Autodesk Inventor part; units mm, degrees
ref_plane "YZ Plane" through (0, 0, 0) normal (1, 0, 0) x (0, 1, 0)
ref_plane "XZ Plane" through (0, 0, 0) normal (0, 1, 0) x (-1, 0, 0)
ref_plane "XY Plane" through (0, 0, 0) normal (0, 0, 1) x (1, 0, 0)
sketch "Sketch1" plane through (0, 0, 0) normal (0, 0, 1) x (1, 0, 0)
  line L0 (22.5, -10) -> (-22.5, -10) construction
  line L1 (-22.5, -10) -> (-22.5, 10) construction
  line L2 (-22.5, 10) -> (22.5, 10) construction
  line L3 (22.5, 10) -> (22.5, -10) construction
  line L4 (22.5, -10) -> (-22.5, 10) construction
  line L5 (-22.5, -10) -> (22.5, 10) construction
  line L6 (-22.5, 13) -> (-22.5, 7) construction
  line L7 (-24.25, 13) -> (-24.25, 7)
  line L8 (-20.75, 7) -> (-20.75, 13)
  arc A0 (-20.75, 13) -> (-24.25, 13) centre (-22.5, 13) ccw
  arc A1 (-24.25, 7) -> (-20.75, 7) centre (-22.5, 7) ccw
  line L9 (-22.5, -13) -> (-22.5, -7) construction
  line L10 (-20.75, -13) -> (-20.75, -7)
  line L11 (-24.25, -7) -> (-24.25, -13)
  arc A2 (-24.25, -13) -> (-20.75, -13) centre (-22.5, -13) ccw
  arc A3 (-20.75, -7) -> (-24.25, -7) centre (-22.5, -7) ccw
  line L12 (22.5, 13) -> (22.5, 7) construction
  line L13 (20.75, 13) -> (20.75, 7)
  line L14 (24.25, 7) -> (24.25, 13)
  arc A4 (24.25, 13) -> (20.75, 13) centre (22.5, 13) ccw
  arc A5 (20.75, 7) -> (24.25, 7) centre (22.5, 7) ccw
  line L15 (22.5, -13) -> (22.5, -7) construction
  line L16 (24.25, -13) -> (24.25, -7)
  line L17 (20.75, -7) -> (20.75, -13)
  arc A6 (20.75, -13) -> (24.25, -13) centre (22.5, -13) ccw
  arc A7 (24.25, -7) -> (20.75, -7) centre (22.5, -7) ccw
  line L18 (26, -16.5) -> (-26, -16.5)
  line L19 (-26, -16.5) -> (-26, 16.5)
  line L20 (-26, 16.5) -> (26, 16.5)
  line L21 (26, 16.5) -> (26, -16.5)
  line L22 (26, -16.5) -> (-26, 16.5) construction
  line L23 (-26, -16.5) -> (26, 16.5) construction
  circle A8 centre (0, 0) radius 6.35
  dimension "d0" = 45
  dimension "d1" = 20
  dimension "d2" = 3.5
  dimension "d3" = 6
  dimension "d4" = 52
  dimension "d5" = 33
  dimension "d6" = 12.7
extrude "Extrusion1" add sketch "Sketch1" along normal blind 4.7625
fillet "Fillet1" radius 2 4 edges at (-26, 16.5, 2.3813) (26, 16.5, 2.3813) (26, -16.5, 2.3813) (-26, -16.5, 2.3813)
properties part number "belt tensioner"
Source: CAD feature listing. Evaluate the final solid. Frame: model axes, mm. A direction names the side the tool comes from. Coordinates: 2 decimals unless noted, no trailing zeros. Loops run counter-clockwise (first coordinate to the right, second up) from the corner with the lowest first, then second, coordinate; pieces in that order, holes last. Notation, with made-up numbers: (75.25, 73) - (104.25, 73) arc R18 ccw to (104.25, 95) - close; hole circle Ø6 at (72, 20). An arc over 180 degrees is marked (long way). One line per question, with ' | ' between items.
1) Line query: line 1 along X through (y, z) = (9.5, 3.6); line 2 along Y through (x, z) = (0, 1.55); line 3 along X through (y, z) = (14, 0.75). Output: solid intervals per line, ascending.
Report:
line 1: x = -26 to -24.25, -20.75 to 20.75, 24.25 to 26 | line 2: y = -16.5 to -6.35, 6.35 to 16.5 | line 3: x = -26 to -23.94, -21.06 to 21.06, 23.94 to 26
2) Section C-C, the plane z = 3.5. Return loops of the section in (x, y), then the cut area to 3 significant figures.
Report:
outline: (-26, -14.5) arc R2 ccw to (-24, -16.5) - (24, -16.5) arc R2 ccw to (26, -14.5) - (26, 14.5) arc R2 ccw to (24, 16.5) - (-24, 16.5) arc R2 ccw to (-26, 14.5) - close; hole (-24.25, -13) arc R1.75 ccw to (-20.75, -13) - (-20.75, -7) arc R1.75 ccw to (-24.25, -7) - close; hole (-24.25, 7) arc R1.75 ccw to (-20.75, 7) - (-20.75, 13) arc R1.75 ccw to (-24.25, 13) - close; hole circle Ø12.7 at (0, 0); hole (20.75, -13) arc R1.75 ccw to (24.25, -13) - (24.25, -7) arc R1.75 ccw to (20.75, -7) - close; hole (20.75, 7) arc R1.75 ccw to (24.25, 7) - (24.25, 13) arc R1.75 ccw to (20.75, 13) - close | area: 1,460 mm²
3) Pull-direction query (X, two-part tool) for faces 3 (the face through (-6, 4, 4.762)), 4 (the face through (20.75, 10, 2)), 5 (the face through (26, 0, 2)); classes: released by +X, released by -X, zero draft, split by the parting line, or undercut.
Report:
face 3: zero draft | face 4: undercut | face 5: released by +X
4) Set-up query: faces 1 (the face through (-24.25, -10, 2)), 2 (the face through (0, -16.5, 2)). Return all of +Z, -Z, +X, -X, +Y, -Y with unobstructed straight access to the full face (end or side cutting, diameter ignored); none if empty.
Report:
face 1: +Z, -Z | face 2: +Z, -Z, +X, -X, -Y
5) Section A-A, the plane x = 22.5. Return loops of the section in (y, z).
Report:
outline: (-16.5, 0) - (-14.75, 0) - (-14.75, 4.76) - (-16.5, 4.76) - close; (-5.25, 0) - (5.25, 0) - (5.25, 4.76) - (-5.25, 4.76) - close; (14.75, 0) - (16.5, 0) - (16.5, 4.76) - (14.75, 4.76) - close
6) Section B-B, the plane y = 0. Return loops of the section in (x, z).
Report:
outline: (-26, 0) - (-6.35, 0) - (-6.35, 4.76) - (-26, 4.76) - close; (6.35, 0) - (26, 0) - (26, 4.76) - (6.35, 4.76) - close
7) Section D-D, the plane y = -9. Return loops of the section in (x, z).
Report:
outline: (-26, 0) - (-24.25, 0) - (-24.25, 4.76) - (-26, 4.76) - close; (-20.75, 0) - (20.75, 0) - (20.75, 4.76) - (-20.75, 4.76) - close; (24.25, 0) - (26, 0) - (26, 4.76) - (24.25, 4.76) - close
